Autodesk Inventor part; units mm, degrees
ref_plane "YZ Plane" through (0, 0, 0) normal (1, 0, 0) x (0, 1, 0)
ref_plane "XZ Plane" through (0, 0, 0) normal (0, 1, 0) x (-1, 0, 0)
ref_plane "XY Plane" through (0, 0, 0) normal (0, 0, 1) x (1, 0, 0)
sketch "Boceto1" plane through (0, 0, 0) normal (0, 0, 1) x (1, 0, 0)
  line L0 (-15, 0) -> (15, 0)
  line L1 (15, 0) -> (15, 5)
  line L2 (15, 5) -> (5, 5)
  line L3 (5, 5) -> (5, 17.5)
  line L4 (5, 17.5) -> (10, 17.5)
  line L5 (10, 17.5) -> (10, 20)
  line L6 (10, 20) -> (-10, 20)
  line L7 (-10, 20) -> (-10, 17.5)
  line L8 (-10, 17.5) -> (-5, 17.5)
  line L9 (-5, 17.5) -> (-5, 5)
  line L10 (-5, 5) -> (-15, 5)
  line L11 (-15, 5) -> (-15, 0)
  line L12 (-15, -10) -> (15, -10)
  point P0 (0, 0)
  point P1 (0, 0)
  point P2 (7.5, 17.5)
  point P3 (10, 5)
  dimension "d6" = 30
  dimension "d7" = 20
  dimension "d8" = 5
  dimension "d9" = 60
  dimension "d10" = 55
  dimension "d11" = 30
  dimension "d12" = 20
revolve "Revolución1" add sketch "Boceto1" angle 360 about axis through (-15, -10, 0) along (1, 0, 0)
properties part number "Rueda polea"
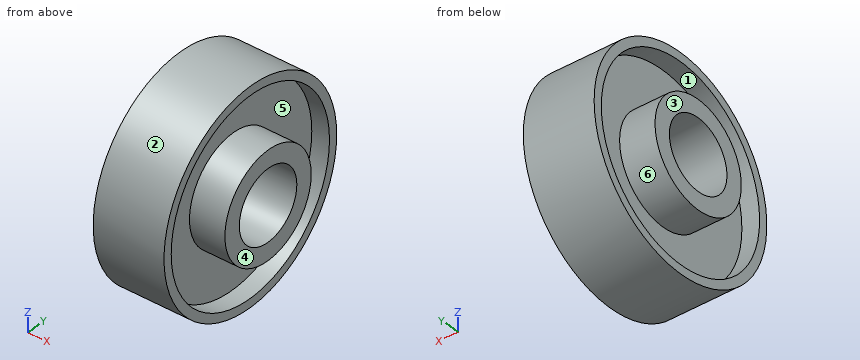
Can you work these out from the model? Positions are in its coordinate system, mm. Face numbers are marked on the shaded views. A direction names the side the tool comes from. Coordinates: 2 decimals unless noted, no trailing zeros. Write each loop counter-clockwise with the first axis right and the second up, starting at its lowest first coordinate (ties: lowest second). Pieces come first, ordered by that corner, then holes. Notation, with made-up numbers: M -40,-28 L 3,-28 A6 cw 3,-20 Z; hole C 49.5,83.5 d5. An arc over 180 degrees is marked long. Write item = value, one per line. Start each with the question number.
Q1. Thinking about a two-plate mould opening in Z: for the marked faces 1, 2 and 3, which applies, released by +Z, released by -Z, zero draft, split by the parting line, or undercut?
Q2. If we section it at C-C, the plane x = -2: Write out the boundary of the cut face in (y, z).
Q3. I'm going to push flat-ended pins straight in: pin 1 (10 mm diameter, centred on x = 12, y = -28, fed in from -Z); pin 2 (1 mm diameter, centred on y = -21, z = 19, fed in from -X); pin 3 (5 mm diameter, centred on x = 2.5, y = -6.5, fed in from +Z). Where does each tip first touch, or does it pass through?
Q4. If we section it at A-A, the plane z = 0: Write out the boundary of the cut face in (x, y), then the cut area to 3 significant figures.
Q5. If I drill on L1, parallel to Z at x = -8.5, y = -15; L2, parallel to Y at x = 8.5, z = -8; L3, parallel to Z at x = -2.25, y = -10, over which ranges is the centre line in solid material (lowest first)? Write a range as [from, to].
Q6. On a 3-axis mill with a long thin cutter (end or side, diameter ignored), from which of +Z, -Z, +X, -X, +Y, -Y can I reach the whole of each face in a straight line? I mean the marked faces 4, 5 and 6. Say none if no direction works.
Q7. If we section it at B-B, the plane y = -5: Write out the boundary of the cut face in (x, z), then the cut area to 3 significant figures.
Q8. If we section it at D-D, the plane y = 11.5: Write out the boundary of the cut face in (x, z), then the cut area to 3 significant figures.
Check sheet entries:
q1.face_1 = undercut
q1.face_2 = split by the parting line
q1.face_3 = zero draft
q2.outline = C -10,0 d60; hole C -10,0 d20
q3.pin_1 = -26.83
q3.pin_2 = -5
q3.pin_3 = 29.98
q4.outline = M -15,-25 L -5,-25 L -5,-37.5 L -10,-37.5 L -10,-40 L 10,-40 L 10,-37.5 L 5,-37.5 L 5,-25 L 15,-25 L 15,-20 L -15,-20 Z; M -15,0 L 15,0 L 15,5 L 5,5 L 5,17.5 L 10,17.5 L 10,20 L -10,20 L -10,17.5 L -5,17.5 L -5,5 L -15,5 Z
q4.area = 650 mm²
q5.L1 = [-29.58, -27.04], [-14.14, -8.66], [8.66, 14.14], [27.04, 29.58]
q5.L2 = [-38.91, -36.31], [-22.69, -16], [-4, 2.69], [16.31, 18.91]
q5.L3 = [-30, -10], [10, 30]
q6.face_4 = +Z, -Z, +X, +Y, -Y
q6.face_5 = +X
q6.face_6 = -X
q7.outline = M -15,-14.14 L -5,-14.14 L -5,-27.04 L -10,-27.04 L -10,-29.58 L 10,-29.58 L 10,-27.04 L 5,-27.04 L 5,-14.14 L 15,-14.14 L 15,-8.66 L -15,-8.66 Z; M -15,8.66 L 15,8.66 L 15,14.14 L 5,14.14 L 5,27.04 L 10,27.04 L 10,29.58 L -10,29.58 L -10,27.04 L -5,27.04 L -5,14.14 L -15,14.14 Z
q7.area = 688 mm²
q8.outline = M -10,-20.92 L 10,-20.92 L 10,-17.15 L 5,-17.15 L 5,17.15 L 10,17.15 L 10,20.92 L -10,20.92 L -10,17.15 L -5,17.15 L -5,-17.15 L -10,-17.15 Z
q8.area = 494 mm²
